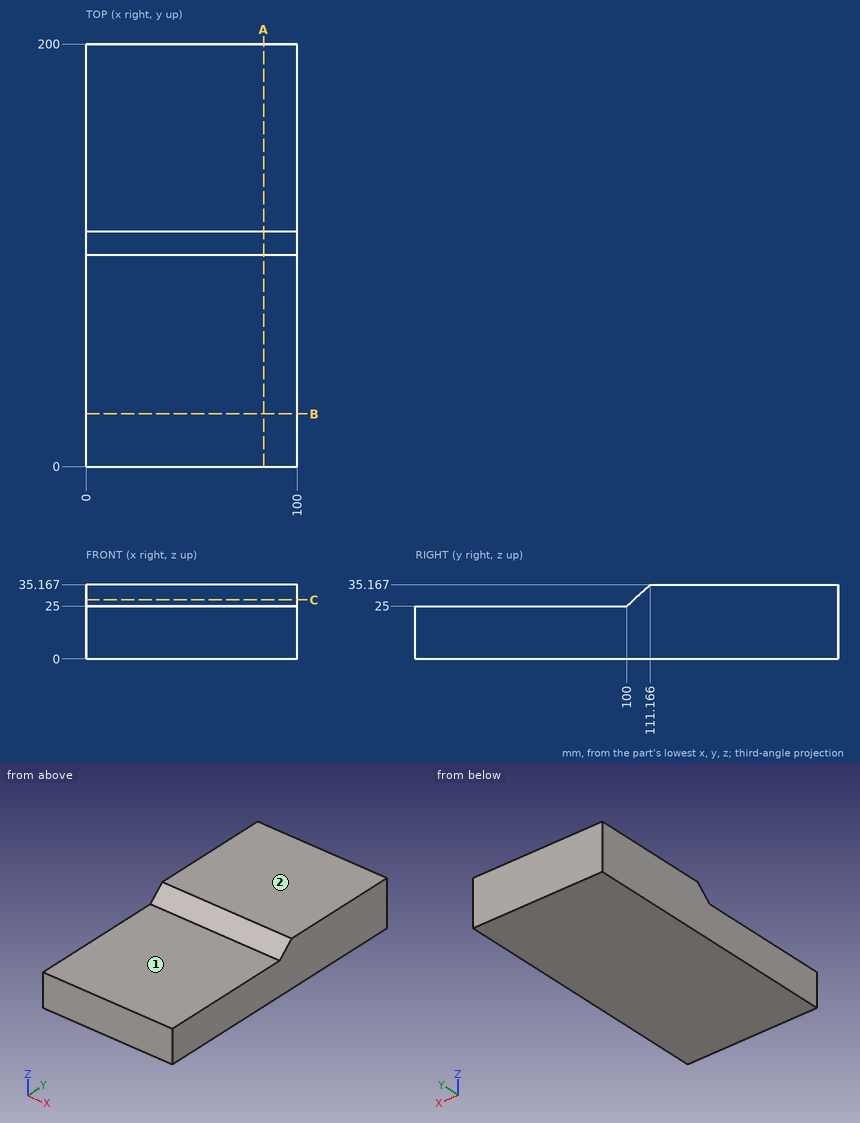
The figure shows three views and two pictorial views of one solid part (mm, origin at its lowest corner). Answer the questions. A direction names the side the tool comes from. Coordinates: 2 decimals unless noted, no trailing zeros. Order: outer loops, then holes, each group sorted by start corner. A loop starts at its lowest first (then second) coordinate and runs counter-clockwise, first axis right, second up.
Q1. Which of the six approach directions +Z, -Z, +X, -X, +Y, -Y give full straight-line access (tool end or side, diameter ignored) to the marked faces 1 and 2?
Q2. Given P1, Ø10, axis at x = 36.5, y = 75, coming from the +Z side; P2, Ø2, axis at x = 89.5, z = 27, coming from the -Y side; P3, Ø6, axis at x = 83, y = 101.5, coming from the +Z side, each flat-ended and moving along its own axis, determine where each tip first touches the part or whether it passes through.
Q3. A cutting plane is placed at B-B, the plane y = 25. Write down the section's boundary in (x, z).
Q4. Consider line 1 (Z direction, x = 95.5, y = 55); line 2 (Y direction, x = 64.5, z = 28) (1 decimal); line 3 (Y direction, x = 13, z = 26). Determine where each line is inside the solid, lowest interval first.
Q5. A cutting plane is placed at C-C, the plane z = 28. Write down the section's boundary in (x, y) (1 decimal), and give its area (3 significant figures).
Q6. A cutting plane is placed at A-A, the plane x = 84. Write down the section's boundary in (y, z), and give its area (3 significant figures).
Answers follow:
1. face 1: +Z, +X, -X, -Y
1. face 2: +Z, +X, -X, +Y, -Y
2. P1: stops at z = 25
2. P2: stops at y = 101.1
2. P3: stops at z = 29.1
3. outline: (0, 0) - (100, 0) - (100, 25) - (0, 25) - close
4. line 1: z = 0 to 25
4. line 2: y = 103.3 to 200
4. line 3: y = 101.1 to 200
5. outline: (0, 103.3) - (100, 103.3) - (100, 200) - (0, 200) - close
5. area: 9,670 mm2
6. outline: (0, 0) - (200, 0) - (200, 35.17) - (111.17, 35.17) - (100, 25) - (0, 25) - close
6. area: 5,960 mm2
